Read the model definition and answer for the solid it produces. Units are mm, in the model's axes. Face numbers are marked on the shaded views. A direction names the side the tool comes from. Coordinates: 2 decimals unless noted, no trailing zeros. Write each loop counter-clockwise with the first axis right and the second up, starting at its lowest first coordinate (ties: lowest second). Pieces come first, ordered by that corner, then holes. Notation, with made-up numbers: (-21.75, 87) - (24.25, 87) arc R10 cw to (24.25, 96) - close; hole circle Ø8 at (21.25, 71.5). An arc over 180 degrees is marked (long way). Use a Markdown table: item, result.
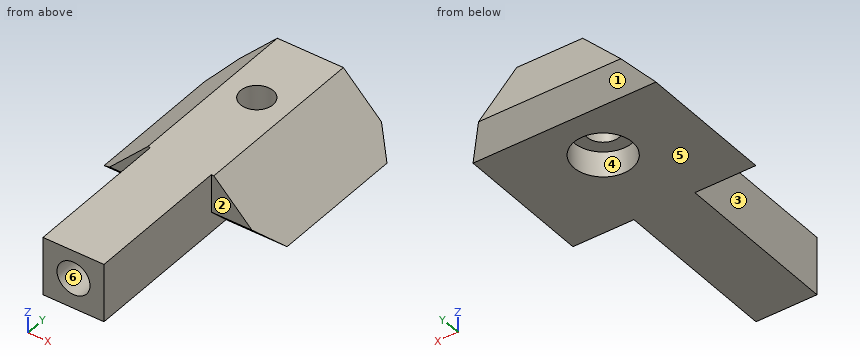
from build123d import *

# Parameters (mm, degrees)
BOSS_EXTRUDE1_DEPTH = 32
CHAMFER1_SIZE       = 2
CUT_EXTRUDE1_DEPTH  = 14.5
CHAMFER2_SIZE       = 2
SKETCH3_R           = 1.625
CUT_EXTRUDE2_DEPTH  = 4
SKETCH4_R           = 1.6
CUT_EXTRUDE3_DEPTH  = 7
SKETCH5_R           = 2.875
CUT_EXTRUDE4_DEPTH  = 2.5
SKETCH6_W           = 9.951006948
SKETCH6_H           = 32
CUT_EXTRUDE5_DEPTH  = 0.25


with BuildPart() as part:
    # Sketch1 → Boss-Extrude1 (new body)
    with BuildSketch(Plane(origin=(0, 0, 0), x_dir=(1, 0, 0), z_dir=(0, 1, 0))):
        Polygon((-16.800646523, 6.80487106), (1.199353477, 6.80487106), (-4.800646523, 0.80487106), (-10.800646523, 0.80487106), align=None)
    extrude(amount=BOSS_EXTRUDE1_DEPTH)

    # Chamfer1
    chamfer1_edges = [part.edges().sort_by_distance(p)[0] for p in [
        (-7.800646523, 32, -6.80487106),
    ]]
    chamfer(chamfer1_edges, length=CHAMFER1_SIZE)

    # Sketch2 → Cut-Extrude1 (cut)
    with BuildSketch(Plane.XZ):
        Polygon((-4.800646523, -0.80487106), (-4.800646523, -6.80487106), (1.199353477, -6.80487106), align=None)
        Polygon((-10.800646523, -0.80487106), (-10.800646523, -6.80487106), (-16.800646523, -6.80487106), align=None)
    extrude(amount=-CUT_EXTRUDE1_DEPTH, mode=Mode.SUBTRACT)

    # Chamfer2
    chamfer2_edges = [part.edges().sort_by_distance(p)[0] for p in [
        (-1.800646523, 14.5, -6.80487106),
        (-13.800646523, 14.5, -6.80487106),
    ]]
    chamfer(chamfer2_edges, length=CHAMFER2_SIZE)

    # Sketch3 → Cut-Extrude2 (cut)
    with BuildSketch(Plane.XZ):
        with Locations((-7.800646523, -3.80487106)):
            Circle(SKETCH3_R)
    extrude(amount=-CUT_EXTRUDE2_DEPTH, mode=Mode.SUBTRACT)

    # Sketch4 → Cut-Extrude3 (cut, through all)
    with BuildSketch(Plane(origin=(0, 0, -6.80487106), x_dir=(-1, 0, 0), z_dir=(0, 0, -1))):
        with Locations((7.800646523, 24.7693)):
            Circle(SKETCH4_R)
    extrude(amount=-CUT_EXTRUDE3_DEPTH, mode=Mode.SUBTRACT)

    # Sketch5 → Cut-Extrude4 (cut)
    with BuildSketch(Plane(origin=(0, 0, -6.80487106), x_dir=(-1, 0, 0), z_dir=(0, 0, -1))):
        with Locations((7.800646523, 24.7693)):
            Circle(SKETCH5_R)
    extrude(amount=-CUT_EXTRUDE4_DEPTH, mode=Mode.SUBTRACT)

    # Sketch6 → Cut-Extrude5 (cut)
    with BuildSketch(Plane.XY.offset(-0.80487106)):
        with Locations((-7.355555637, 16)):
            Rectangle(SKETCH6_W, SKETCH6_H)
    extrude(amount=-CUT_EXTRUDE5_DEPTH, mode=Mode.SUBTRACT)


solid = part.part
(1) A cutting plane is placed at D-D, the plane x = -11.75. Write down the section's boundary in (y, z).
Report:
| item | result |
|---|---|
| outline | (14.5, -4.8) - (16.5, -6.8) - (30, -6.8) - (32, -4.8) - (32, -1.75) - (14.5, -1.75) - close |
(2) Each of these flat-tipped pins is pushed along its axis until it touches: P1, Ø3, axis at y = 14, z = -1.5, coming from the +X side; P2, Ø2.5, axis at x = -7.8, y = 24.77, coming from the +Z side; P3, Ø3, axis at x = -8, y = 26, coming from the -Z side; P4, Ø1, axis at y = 16, z = -2, coming from the +X side. Where does it stop, or does it pass through?
Report:
| item | result |
|---|---|
| P1 | stops at x = -2.69 |
| P2 | passes through |
| P3 | stops at z = -4.3 |
| P4 | stops at x = -3.11 |
(3) Straight lines are drawn through the part: L1, parallel to X at y = 3.5, z = -1.9; L2, parallel to Z at x = -10.5, y = 24; L3, parallel to X at y = 25, z = -4.35. For each, find the intervals that lie inside material, in ascending order.
Report:
| item | result |
|---|---|
| L1 | x = -10.8 to -4.8 |
| L2 | z = -4.3 to -1.05 |
| L3 | x = -14.35 to -10.67, -4.93 to -1.26 |
(4) A cutting plane is placed at A-A, the plane x = -8. Write down the section's boundary in (y, z), and give its area (3 significant figures).
Report:
| item | result |
|---|---|
| outline | (0, -6.8) - (21.9, -6.8) - (21.9, -4.3) - (23.18, -4.3) - (23.18, -1.05) - (0, -1.05) - (0, -2.19) - (4, -2.19) - (4, -5.42) - (0, -5.42) - close; (26.36, -4.3) - (27.64, -4.3) - (27.64, -6.8) - (30, -6.8) - (32, -4.8) - (32, -1.05) - (26.36, -1.05) - close |
| area | 144 mm² |
(5) A cutting plane is placed at B-B, the plane z = -3.4. Write down the section's boundary in (x, y).
Report:
| item | result |
|---|---|
| outline | (-13.4, 14.5) - (-10.8, 14.5) - (-10.8, 0) - (-9.37, 0) - (-9.37, 4) - (-6.23, 4) - (-6.23, 0) - (-4.8, 0) - (-4.8, 14.5) - (-2.21, 14.5) - (-2.21, 32) - (-13.4, 32) - close; hole circle Ø3.2 at (-7.8, 24.77) |
(6) A cutting plane is placed at C-C, the plane y = 15. Write down the section's boundary in (x, z).
Report:
| item | result |
|---|---|
| outline | (-15.3, -5.3) - (-10.8, -5.3) - (-10.8, -6.8) - (-4.8, -6.8) - (-4.8, -5.3) - (-0.3, -5.3) - (-4.55, -1.05) - (-11.05, -1.05) - close |
(7) The mould has two halves that part along X. Classify the marked faces 3, 4, 5 and 6: pulls with the +X half, pulls with the -X half, needs draft (parallel to the pull), parting line crosses it, or undercut.
Report:
| item | result |
|---|---|
| face 3 | pulls with the -X half |
| face 4 | undercut |
| face 5 | needs draft |
| face 6 | undercut |
(8) For the marked faces 1 and 2, determine the directions among +Z, -Z, +X, -X, +Y, -Y from which every point of the face is accessible in a straight line to the end or side of a thin tool.
Report:
| item | result |
|---|---|
| face 1 | -Z, +X, -X, +Y |
| face 2 | +Z, -Z, +X, -Y |
